from build123d import *

# Parameters (mm, degrees)
T_LE_DE_BASE_PLI_E1_DEPTH = 160
ENL_V_MAT_EXTRU_1_REACH   = 277.896
ESQUISSE2_W               = 39.08587988
ESQUISSE2_H               = 15


# Read off the part's stored shape, not the designer's step: Tôle de base pliée1
with BuildPart() as part:
    # Tôle de base pliée1 outline → Tôle de base pliée1 (new body)
    with BuildSketch(Plane(origin=(0, 0, 0), x_dir=(1, 0, 0), z_dir=(0, 1, 0))):
        with BuildLine():
            Line((155, -53.5), (74.5, -53.5))
            Line((74.5, -53.5), (74.5, -54.5))
            Line((74.5, -54.5), (155, -54.5))
            ThreePointArc((155, -54.5), (161.717514421, -51.717514421), (164.5, -45))
            Line((164.5, -45), (164.5, 61))
            ThreePointArc((164.5, 61), (163.474873734, 63.474873734), (161, 64.5))
            Line((161, 64.5), (98.72391992, 64.5))
            ThreePointArc((98.72391992, 64.5), (93.97391992, 63.227241336), (90.496678584, 59.75))
            Line((90.496678584, 59.75), (58.453738644, 4.25))
            ThreePointArc((58.453738644, 4.25), (55.342522712, 1.138784068), (51.092522712, 0))
            Line((51.092522712, 0), (-51.092522712, 0))
            ThreePointArc((-51.092522712, 0), (-55.342522712, 1.138784068), (-58.453738644, 4.25))
            Line((-58.453738644, 4.25), (-90.496678584, 59.75))
            ThreePointArc((-90.496678584, 59.75), (-93.97391992, 63.227241336), (-98.72391992, 64.5))
            Line((-98.72391992, 64.5), (-161, 64.5))
            ThreePointArc((-161, 64.5), (-163.474873734, 63.474873734), (-164.5, 61))
            Line((-164.5, 61), (-164.5, -45))
            ThreePointArc((-164.5, -45), (-161.717514421, -51.717514421), (-155, -54.5))
            Line((-155, -54.5), (-74.5, -54.5))
            Line((-74.5, -54.5), (-74.5, -53.5))
            Line((-74.5, -53.5), (-155, -53.5))
            ThreePointArc((-155, -53.5), (-161.01040764, -51.01040764), (-163.5, -45))
            Line((-163.5, -45), (-163.5, 61))
            ThreePointArc((-163.5, 61), (-162.767766953, 62.767766953), (-161, 63.5))
            Line((-161, 63.5), (-98.72391992, 63.5))
            ThreePointArc((-98.72391992, 63.5), (-94.47391992, 62.361215932), (-91.362703988, 59.25))
            Line((-91.362703988, 59.25), (-59.319764048, 3.75))
            ThreePointArc((-59.319764048, 3.75), (-55.842522712, 0.272758664), (-51.092522712, -1))
            Line((-51.092522712, -1), (51.092522712, -1))
            ThreePointArc((51.092522712, -1), (55.842522712, 0.272758664), (59.319764048, 3.75))
            Line((59.319764048, 3.75), (91.362703988, 59.25))
            ThreePointArc((91.362703988, 59.25), (94.47391992, 62.361215932), (98.72391992, 63.5))
            Line((98.72391992, 63.5), (161, 63.5))
            ThreePointArc((161, 63.5), (162.767766953, 62.767766953), (163.5, 61))
            Line((163.5, 61), (163.5, -45))
            ThreePointArc((163.5, -45), (161.01040764, -51.01040764), (155, -53.5))
        make_face()
    extrude(amount=T_LE_DE_BASE_PLI_E1_DEPTH)

    # Esquisse2 → Enlèv. mat.-Extru.1 (cut, up to next)
    with BuildSketch(Plane(origin=(42, 0, 24.248711306), x_dir=(-0.4999999999999975, 0, 0.86602540378444), z_dir=(-0.86602540378444, 0, -0.4999999999999975)), mode=Mode.PRIVATE) as enl_v_mat_extru_1_sk1:
        with Locations((-62.450417228, 152.5)):
            Rectangle(ESQUISSE2_W, ESQUISSE2_H)
    enl_v_mat_extru_1_tool1 = extrude(enl_v_mat_extru_1_sk1.sketch, amount=-ENL_V_MAT_EXTRU_1_REACH, mode=Mode.PRIVATE) & part.part
    enl_v_mat_extru_1 = enl_v_mat_extru_1_tool1.solids().sort_by_distance((73.225209, 152.5, -29.834936))[0]
    add(enl_v_mat_extru_1, mode=Mode.SUBTRACT)

    # Symétrie1: Enlèv. mat.-Extru.1 across plane
    add(enl_v_mat_extru_1.mirror(Plane(origin=(0, 0, 0), x_dir=(0, 0, 1), z_dir=(1, 0, 0))), mode=Mode.SUBTRACT)


solid = part.part
Can you work these out from the model? Positions are in its coordinate system, mm. A direction names the side the tool comes from. Coordinates: 2 decimals unless noted, no trailing zeros. Write each loop counter-clockwise with the first axis right and the second up, starting at its lowest first coordinate (ties: lowest second). Pieces come first, ordered by that corner, then holes.
Q1. Which directions (+Z, -Z, +X, -X, +Y, -Y) give clear straight access to the entire face, cutting with the end or side of a thin tool? Please do faces 4 (the face through (-114, 79, 53.5)), 5 (the face through (55.4, 78.88, -1.17)), 6 (the face through (55.782, 78.88, -0.238)).
Results found:
face 4: +Y, -Y
face 5: -Z, +Y, -Y
face 6: +Z, +Y, -Y
Q2. Imagine slicing it at C-C, the plane z = -34.5. List the corners of the cut face in (x, y) for me, plus the area to 3 significant figures.
Results found:
outline: (-164.5, 0) - (-163.5, 0) - (-163.5, 160) - (-164.5, 160) - close; (-77.07, 0) - (-75.92, 0) - (-75.92, 145) - (-77.07, 145) - close; (75.92, 0) - (77.07, 0) - (77.07, 145) - (75.92, 145) - close; (163.5, 0) - (164.5, 0) - (164.5, 160) - (163.5, 160) - close
area: 655 mm2
Q3. Imagine slicing it at D-D, the plane x = -17. List the corners of the cut face in (y, z) for me, plus the area to 3 significant figures.
Results found:
outline: (0, 0) - (160, 0) - (160, 1) - (0, 1) - close
area: 160 mm2
Q4. Please list where these lines run through material, in increasing order: L1, parallel to X at y = 10, z = 35; L2, parallel to Z at x = -151, y = 82; L3, parallel to X at y = 93.5, z = -15.
Results found:
L1: x = -164.5 to -163.5, 163.5 to 164.5
L2: z = -64.5 to -63.5, 53.5 to 54.5
L3: x = -164.5 to -163.5, -65.81 to -64.66, 64.66 to 65.81, 163.5 to 164.5
Q5. For P1, Ø12, axis at x = -93, y = 56.5, coming from the -Z side; P2, Ø6, axis at x = 73, z = -25.5, coming from the +Y side, each with a flat end and sliding along its axis, tell me the tip position at first contact or that it passes through.
Results found:
P1: stops at z = -64.5
P2: stops at y = 145
Q6. Imagine slicing it at A-A, the plane z = 16. List the corners of the cut face in (x, y) for me, plus the area to 3 significant figures.
Results found:
outline: (-164.5, 0) - (-163.5, 0) - (-163.5, 160) - (-164.5, 160) - close; (163.5, 0) - (164.5, 0) - (164.5, 160) - (163.5, 160) - close
area: 320 mm2
Q7. Imagine slicing it at B-B, the plane x = -119. List the corners of the cut face in (y, z) for me, plus the area to 3 significant figures.
Results found:
outline: (0, -64.5) - (160, -64.5) - (160, -63.5) - (0, -63.5) - close; (0, 53.5) - (160, 53.5) - (160, 54.5) - (0, 54.5) - close
area: 320 mm2
Q8. If we mould it in two halves opening along X, with no side actions, what happens to faces 1 (the face through (115, 79, 53.5)), 2 (the face through (114, 79, 54.5)), 3 (the face through (164.5, 79, -7))? For each: +X half, -X half, draft (parallel to the pull), parting line (faces both ways), or undercut.
Results found:
face 1: undercut
face 2: draft
face 3: +X half
